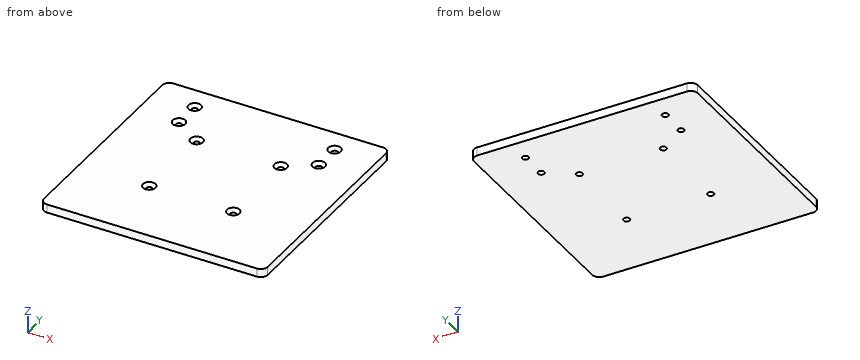
Solid Edge part; units mm, degrees
sketch "Sketch1" plane through (60.3162, 60.3162, 0) normal (0, 0, 1) x (1, 0, 0)
  line L0 (-140.3162, -140.3162) -> (19.6838, -140.3162)
  line L1 (19.6838, -140.3162) -> (19.6838, 19.6838)
  line L2 (19.6838, 19.6838) -> (-140.3162, 19.6838)
  line L3 (-140.3162, 19.6838) -> (-140.3162, -140.3162)
  dimension "D1" = 19.6838
  dimension "D2" = 19.6838
extrude "Protrusion1" add sketch "Sketch1" along normal mid plane 6
fillet "Verrundung_1" radius 5 4 edges at (-80, 80, 0) (80, 80, 0) (80, -80, 0) (-80, -80, 0)
hole "Bohrung_1" at (30.052, 30.052, 3) direction (0, 0, -1) diameter 4.5 end up to next countersink diameter 9 countersink angle 90
pattern_circular "Pattern1" count 4 over 360 about axis through (0, 0, 3) along (0, 0, 1) of "Bohrung_1"
hole "Bohrung_2" at (-50, 63, 3) direction (0, 0, -1) diameter 4.5 end up to next countersink diameter 9 countersink angle 90
hole "Hole1" at (-50, 43, 3) direction (0, 0, -1) diameter 4.5 end up to next countersink diameter 9 countersink angle 90
mirror "Mirror1" about plane through (0, 5.5244, 5.5244) normal (1, 0, 0) of "Bohrung_2", "Hole1"
properties material "Aluminium, 1060"
The model under review builds one solid part; all positions refer to its coordinate system, in mm. Round coordinates to 2 decimals unless told otherwise and drop trailing zeros. Loops run counter-clockwise (first coordinate to the right, second up) from the corner with the lowest first, then second, coordinate; pieces in that order, holes last. Notation, with made-up numbers: M 56.5,3.25 L 108.5,3.25 A23 ccw 108.5,31.25 Z; hole C -38,-13 d5. An arc over 180 degrees is marked long. Answer as CSV lines item,"result". Start each with the question number.
Item 1: Insertion check: P1, Ø6, axis at x = -30.052, y = -30.052, coming from the +Z side; P2, Ø7, axis at x = 50, y = 63, coming from the +Z side. Each pin has a flat end and moves straight along its axis. Give the tip position at first contact, or say it passes through.
Item 2: Consider section B-B (y = 43). Write out the cut boundary in (x, z).
Item 3: Consider section A-A (x = -50). Write out the cut boundary in (y, z).
Item 4: Wall thickness on line 1 (Y direction, x = -50, z = -0.7); line 2 (Y direction, x = -30.5, z = 0.3); line 3 (X direction, y = 63, z = -1.2): over which ranges is each line inside the solid? List them lowest first. Write a range as [from, to].
Answer:
1,P1,"stops at z = 1.5"
1,P2,"stops at z = 2"
2,outline,"M -80,-3 L -52.25,-3 L -52.25,0.75 L -54.5,3 L -80,3 Z; M -47.75,-3 L 47.75,-3 L 47.75,0.75 L 45.5,3 L -45.5,3 L -47.75,0.75 Z; M 52.25,-3 L 80,-3 L 80,3 L 54.5,3 L 52.25,0.75 Z"
3,outline,"M -80,-3 L 40.75,-3 L 40.75,0.75 L 38.5,3 L -80,3 Z; M 45.25,-3 L 60.75,-3 L 60.75,0.75 L 58.5,3 L 47.5,3 L 45.25,0.75 Z; M 65.25,-3 L 80,-3 L 80,3 L 67.5,3 L 65.25,0.75 Z"
4,line 1,"y = [-80, 40.75], [45.25, 60.75], [65.25, 80]"
4,line 2,"y = [-80, -32.26], [-27.85, 27.85], [32.26, 80]"
4,line 3,"x = [-80, -52.25], [-47.75, 47.75], [52.25, 80]"
